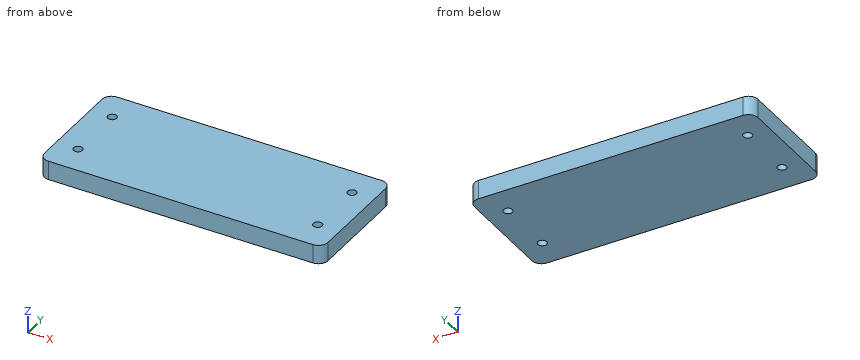
from build123d import *

# Parameters (mm, degrees)
SKETCH_W     = 120
SKETCH_H     = 50
PAD_DEPTH    = 8
SKETCH001_R  = 1.875
POCKET_DEPTH = 8.001
FILLET_R     = 4


with BuildPart() as part:
    # Sketch → Pad (new body)
    with BuildSketch(Plane.XY):
        Rectangle(SKETCH_W, SKETCH_H)
    extrude(amount=PAD_DEPTH)

    # Sketch001 (on Face6 of Pad) → Pocket (cut, through all)
    with BuildSketch(Plane.XY.offset(8)):
        with Locations((-50.75, 12.5)):
            Circle(SKETCH001_R)
        with Locations((50.75, 12.5)):
            Circle(SKETCH001_R)
        with Locations((-50.75, -12.5)):
            Circle(SKETCH001_R)
        with Locations((50.75, -12.5)):
            Circle(SKETCH001_R)
    extrude(amount=-POCKET_DEPTH, mode=Mode.SUBTRACT)

    # Fillet
    fillet_edges = [part.edges().sort_by_distance(p)[0] for p in [
        (-60, 25, 4),
        (-60, -25, 4),
        (60, -25, 4),
        (60, 25, 4),
    ]]
    fillet(fillet_edges, radius=FILLET_R)


solid = part.part
Here's how the part is built. I have some questions about the finished solid (model axes, mm). Round coordinates to 2 decimals unless told otherwise and drop trailing zeros. Loops run counter-clockwise (first coordinate to the right, second up) from the corner with the lowest first, then second, coordinate; pieces in that order, holes last. Notation, with made-up numbers: M 87.5,17 L 145.5,17 A15 ccw 145.5,46 Z; hole C 55.5,8 d10. An arc over 180 degrees is marked long. Write each question's results on one line, items separated by ' | '. Start each with the question number.
(1) I want a section at B-B (y = -12.5). Please give me the cut outline in (x, z) (3 decimals).
(2) If I drill on probe 1 along Y at (x, z) = (-50.75, 6.75) (3 decimals); probe 2 along X at (y, z) = (13, 7); probe 3 along Y at (x, z) = (50, 6.5), over which ranges is the centre line in solid material (lowest first)? Write a range as from..to.
(3) Will this pin go through, and if not, where does the flat tip stop? P1, Ø3, axis at x = -50.75, y = 12.5, coming from the +Z side.
(4) I want a section at A-A (x = 50.75). Please give me the cut outline in (y, z) (3 decimals).
Solved:
1) outline: M -60,0 L -52.625,0 L -52.625,8 L -60,8 Z; M -48.875,0 L 48.875,0 L 48.875,8 L -48.875,8 Z; M 52.625,0 L 60,0 L 60,8 L 52.625,8 Z
2) probe 1: y = -25..-14.375, -10.625..10.625, 14.375..25 | probe 2: x = -60..-52.56, -48.94..48.94, 52.56..60 | probe 3: y = -25..-14.22, -10.78..10.78, 14.22..25
3) P1: passes through
4) outline: M -25,0 L -14.375,0 L -14.375,8 L -25,8 Z; M -10.625,0 L 10.625,0 L 10.625,8 L -10.625,8 Z; M 14.375,0 L 25,0 L 25,8 L 14.375,8 Z
